Part model, mm, in its own coordinate system. A direction names the side the tool comes from. Round coordinates to 2 decimals unless told otherwise and drop trailing zeros. Loops run counter-clockwise (first coordinate to the right, second up) from the corner with the lowest first, then second, coordinate; pieces in that order, holes last. Notation, with made-up numbers: (82, 89.25) -> (101, 89.25) arc R29 cw to (101, 121.25) -> close; hole circle Ø4 at (51.5, 33.25). An arc over 180 degrees is marked (long way). Use a Markdown table: item, result. Add a question column.
Item 1: Flat gauge pins, fed straight in: pin 1 (1.5 mm diameter, centred on y = -1, z = -6.5, fed in from +X); pin 2 (6 mm diameter, centred on x = -9, z = -7, fed in from -Y); pin 3 (1.5 mm diameter, centred on y = 2.5, z = 0, fed in from -X); pin 4 (10 mm diameter, centred on x = 1.5, z = 0, fed in from -Y). Where does each tip first touch, or does it go through?
Item 2: Which spindle directions (+Z, -Z, +X, -X, +Y, -Y) get a long thin tool onto all of the face, cutting with end or side? Do faces 1 (the face through (10.902, -0.018, 3.433)), 2 (the face through (-0.74, -3.44, 0.68)), 3 (the face through (-0.74, 3.42, 0.68)). Say none if no direction does.
Item 3: Cut at B-B, the plane x = 0. List the corners of the cut face in (y, z), plus the area to 3 significant figures.
Item 4: Cut at D-D, the plane y = 2. List the corners of the cut face in (x, z).
Item 5: Probe line 1 (Y direction, x = 5.5, z = -4); line 2 (Z direction, x = -0.25, y = 0.25); line 3 (X direction, y = -0.25, z = -9). List the from-to ranges inside material, lowest first. Write a range as [from, to].
Item 6: Cut at C-C, the plane y = -3.25. List the corners of the cut face in (x, z), plus the area to 3 significant figures.
Item 7: Cut at A-A, the plane z = 0. List the corners of the cut face in (x, y).
```python
from build123d import *

# Parameters (mm, degrees)
F0_R          = 1.0033
F1_DEPTH      = 4.318
F1_DEPTH_BACK = 4.318
F0_R_2        = 11.43
F2_DEPTH      = 2.54
F2_DEPTH_BACK = 2.54
F3_R          = 1.27


with BuildPart() as f1:
    # F0 (on Front) → F1 (new body, two sides)
    with BuildSketch(Plane.XZ) as f1_sk:
        Circle(F0_R)
    extrude(amount=F1_DEPTH)
    extrude(f1_sk.sketch, amount=-F1_DEPTH_BACK)

    # F0 (on Front) → F2 (join, two sides)
    with BuildSketch(Plane.XZ) as f2_sk:
        Circle(F0_R_2)
        Circle(F0_R, mode=Mode.SUBTRACT)
    extrude(amount=F2_DEPTH)
    extrude(f2_sk.sketch, amount=-F2_DEPTH_BACK)

    # F3
    f3_edges = [f1.edges().sort_by_distance(p)[0] for p in [
        (-11.43, -2.54, 0),
        (-11.43, 2.54, 0),
    ]]
    fillet(f3_edges, radius=F3_R)


solid = f1.part
```
A:
| question | item | result |
|---|---|---|
| 1 | pin 1 | stops at x = 9.88 |
| 1 | pin 2 | stops at y = -2.54 |
| 1 | pin 3 | stops at x = -11.34 |
| 1 | pin 4 | stops at y = -4.32 |
| 2 | face 1 | +Y, -Y |
| 2 | face 2 | -Y |
| 2 | face 3 | +Y |
| 3 | outline | (-4.32, -1) -> (-2.54, -1) -> (-2.54, -10.16) arc R1.27 ccw to (-1.27, -11.43) -> (1.27, -11.43) arc R1.27 ccw to (2.54, -10.16) -> (2.54, -1) -> (4.32, -1) -> (4.32, 1) -> (2.54, 1) -> (2.54, 10.16) arc R1.27 ccw to (1.27, 11.43) -> (-1.27, 11.43) arc R1.27 ccw to (-2.54, 10.16) -> (-2.54, 1) -> (-4.32, 1) -> close |
| 3 | area | 122 mm^2 |
| 4 | outline | circle Ø22.4 at (0, 0) |
| 5 | line 1 | y = [-2.54, 2.54] |
| 5 | line 2 | z = [-11.43, 11.43] |
| 5 | line 3 | x = [-7.05, 7.05] |
| 6 | outline | circle Ø2.01 at (0, 0) |
| 6 | area | 3.16 mm^2 |
| 7 | outline | (-11.43, -1.27) arc R1.27 ccw to (-10.16, -2.54) -> (-1, -2.54) -> (-1, -4.32) -> (1, -4.32) -> (1, -2.54) -> (10.16, -2.54) arc R1.27 ccw to (11.43, -1.27) -> (11.43, 1.27) arc R1.27 ccw to (10.16, 2.54) -> (1, 2.54) -> (1, 4.32) -> (-1, 4.32) -> (-1, 2.54) -> (-10.16, 2.54) arc R1.27 ccw to (-11.43, 1.27) -> close |
